Source: CAD feature listing. Evaluate the final solid. Frame: model axes, mm. A direction names the side the tool comes from. Give positions to 0.01 mm unless a question says otherwise; leave off trailing zeros. Write each loop counter-clockwise with the first axis right and the second up, starting at its lowest first coordinate (ties: lowest second). Pieces come first, ordered by that corner, then holes. Notation, with made-up numbers: (-27.75, 39.5) -> (-7.75, 39.5) arc R30 ccw to (-7.75, 62.5) -> close; hole circle Ø3 at (48, 39.25). An arc over 180 degrees is marked (long way). Write item = value, one per line.
from build123d import *

# Parameters (mm, degrees)
BOSS_EXTRUDE1_DEPTH = 3.175
SKETCH4_W           = 31.75
SKETCH4_H           = 3.175
BOSS_EXTRUDE2_DEPTH = 27.94
SKETCH5_R           = 1.5875
CUT_EXTRUDE2_DEPTH  = 48.204039552
SKETCH6_R           = 1.15
CUT_EXTRUDE3_DEPTH  = 38.357217843


with BuildPart() as part:
    # Sketch1 → Boss-Extrude1 (new body)
    with BuildSketch(Plane.XY):
        with BuildLine():
            ThreePointArc((15.875, 0), (0, 15.875), (-15.875, 0))
            Line((-15.875, 0), (15.875, 0))
        make_face()
        with BuildLine():
            ThreePointArc((15.875, 0), (0, -15.875), (-15.875, 0))
            Line((-15.875, 0), (-15.875, -19.05))
            Line((-15.875, -19.05), (15.875, -19.05))
            Line((15.875, -19.05), (15.875, 0))
        make_face()
        with BuildLine():
            Line((15.875, 0), (-15.875, 0))
            ThreePointArc((-15.875, 0), (0, -15.875), (15.875, 0))
        make_face()
    extrude(amount=BOSS_EXTRUDE1_DEPTH)

    # Sketch4 → Boss-Extrude2 (add)
    with BuildSketch(Plane.XY.offset(3.175)):
        with Locations((0, -17.4625)):
            Rectangle(SKETCH4_W, SKETCH4_H)
    extrude(amount=BOSS_EXTRUDE2_DEPTH)

    # Sketch5 → Cut-Extrude2 (cut, through all)
    with BuildSketch(Plane(origin=(0, -15.875, 0), x_dir=(1, 0, 0), z_dir=(0, 1, 0))):
        with Locations(Location((-9.525, -24.765, 0), (0, 0, 270))):
            Circle(SKETCH5_R)
        with Locations(Location((9.525, -24.765, 0), (0, 0, 90))):
            Circle(SKETCH5_R)
    extrude(amount=-CUT_EXTRUDE2_DEPTH, mode=Mode.SUBTRACT)

    # Sketch6 → Cut-Extrude3 (cut, through all)
    with BuildSketch(Plane.XY.offset(3.175)):
        Circle(SKETCH6_R)
    extrude(amount=-CUT_EXTRUDE3_DEPTH, mode=Mode.SUBTRACT)


solid = part.part
(1) Access query for faces 1 (the face through (-15.875, -17, 11)), 2 (the face through (0, -15.875, 17)). Directions: +Z, -Z, +X, -X, +Y, -Y. A direction counts if a zero-diameter tool reaches every point of the face in a straight line with its end or side. Return the directions, or none.
Values follow:
face_1 = +Z, -Z, -X, +Y, -Y
face_2 = +Z, +X, -X, +Y
(2) Section query D-D (z = 11.5). Return loops of the section in (x, y) (3 decimals), plus the area to 3 significant figures.
Values follow:
outline = (-15.875, -19.05) -> (15.875, -19.05) -> (15.875, -15.875) -> (-15.875, -15.875) -> close
area = 101 mm2
(3) Material intervals for line 1 (Y direction, x = -7.5, z = 27.5) (3 decimals); line 2 (Z direction, x = -4.5, y = -13) (3 decimals); line 3 (Y direction, x = -8.5, z = 3), sorted ascending.
Values follow:
line_1 = -19.05 to -15.875
line_2 = 0 to 3.175
line_3 = -19.05 to 13.41
(4) First-contact query: pin 1 (5 mm diameter, centred on x = -1, z = 6.5, fed in from +Y) (3 decimals); pin 2 (1.5 mm diameter, centred on x = -10.5, y = -12.5, fed in from +Z) (3 decimals). Flat tips, straight axial feed; report the tip coordinate or a pass-through.
Values follow:
pin_1 = -15.875
pin_2 = 3.175
(5) Section query C-C (y = -0.5). Return loops of the section in (x, z) (3 decimals).
Values follow:
outline = (-15.875, 0) -> (-1.036, 0) -> (-1.036, 3.175) -> (-15.875, 3.175) -> close; (1.036, 0) -> (15.875, 0) -> (15.875, 3.175) -> (1.036, 3.175) -> close
(6) Section query A-A (x = 0). Return loops of the section in (y, z) (3 decimals), plus the area to 3 significant figures.
Values follow:
outline = (-19.05, 0) -> (-1.15, 0) -> (-1.15, 3.175) -> (-15.875, 3.175) -> (-15.875, 31.115) -> (-19.05, 31.115) -> close; (1.15, 0) -> (15.875, 0) -> (15.875, 3.175) -> (1.15, 3.175) -> close
area = 192 mm2
(7) Section query B-B (z = 24). Return loops of the section in (x, y) (3 decimals).
Values follow:
outline = (-15.875, -19.05) -> (-10.916, -19.05) -> (-10.916, -15.875) -> (-15.875, -15.875) -> close; (-8.134, -19.05) -> (8.134, -19.05) -> (8.134, -15.875) -> (-8.134, -15.875) -> close; (10.916, -19.05) -> (15.875, -19.05) -> (15.875, -15.875) -> (10.916, -15.875) -> close
(8) Pull-direction query (X, two-part tool) for faces 3 (the face through (0, -19.05, 15)), 4 (the face through (-0.91, -0.7, 1.61)), 5 (the face through (9.05, -17.44, 23.25)), 6 (the face through (0.35, 15.87, 1.57)); classes: pulls with the +X half, pulls with the -X half, needs draft (parallel to the pull), parting line crosses it, or undercut.
Values follow:
face_3 = needs draft
face_4 = undercut
face_5 = undercut
face_6 = parting line crosses it
